```python
from build123d import *

# Parameters (mm, degrees)
EXTRUDE_THIN1_DEPTH          = 10
BOSS_EXTRUDE1_DEPTH          = 2
SKETCH2_W                    = 25.834060226
SKETCH2_H                    = 7.264687176
SKETCH2_W_2                  = 26.707196626
SKETCH2_H_2                  = 6.244092899
CUT_EXTRUDE1_DEPTH           = 92.75076294
SKETCH3_R                    = 4.9
BOSS_EXTRUDE2_DEPTH          = 10
FILLET1_START                = 34.65
FILLET1_DEPTH                = 9.35
FILLET2_R                    = 2
CUT_EXTRUDE2_DEPTH           = 106.894440364
CUT_EXTRUDE2_DEPTH_BACK      = 106.894440364
SKETCH5_R                    = 19.1
SKETCH6_R                    = 2.6162
CUT_EXTRUDE3_DEPTH           = 5
CUT_EXTRUDE3_DRAFT           = -8
CUT_EXTRUDE3_PROFILE_2_DEPTH = 5
CUT_EXTRUDE3_PROFILE_2_DRAFT = -8
CUT_EXTRUDE3_PROFILE_3_DEPTH = 5
CUT_EXTRUDE3_PROFILE_3_DRAFT = -8
CUT_EXTRUDE3_PROFILE_4_DEPTH = 5
CUT_EXTRUDE3_PROFILE_4_DRAFT = -8
SKETCH7_R                    = 2.3495
CUT_EXTRUDE4_DEPTH           = 98.440289419


with BuildPart() as part:
    # Sketch1 → Extrude-Thin1 (new body)
    with BuildSketch(Plane(origin=(0, 32.65, 0), x_dir=(1, 0, 0), z_dir=(0, 1, 0))):
        with BuildLine():
            Line((-69.55, 47.05), (-69.55, -47.05))
            ThreePointArc((-69.55, -47.05), (-66.049926035, -55.499926035), (-57.6, -59))
            Line((-57.6, -59), (-30.4, -59))
            ThreePointArc((-30.4, -59), (-21.950073965, -55.499926035), (-18.45, -47.05))
            Line((-18.45, -47.05), (-18.45, 47.05))
            ThreePointArc((-18.45, 47.05), (-21.950073965, 55.499926035), (-30.4, 59))
            Line((-30.4, 59), (-57.6, 59))
            ThreePointArc((-57.6, 59), (-66.049926035, 55.499926035), (-69.55, 47.05))
        make_face()
        with BuildLine():
            Line((-67.05, 47.05), (-67.05, -47.05))
            ThreePointArc((-67.05, -47.05), (-64.282159082, -53.732159082), (-57.6, -56.5))
            Line((-57.6, -56.5), (-30.4, -56.5))
            ThreePointArc((-30.4, -56.5), (-23.717840918, -53.732159082), (-20.95, -47.05))
            Line((-20.95, -47.05), (-20.95, 47.05))
            ThreePointArc((-20.95, 47.05), (-23.717840918, 53.732159082), (-30.4, 56.5))
            Line((-30.4, 56.5), (-57.6, 56.5))
            ThreePointArc((-57.6, 56.5), (-64.282159082, 53.732159082), (-67.05, 47.05))
        make_face(mode=Mode.SUBTRACT)
    extrude(amount=EXTRUDE_THIN1_DEPTH)

    # Sketch1<2> → Boss-Extrude1 (add)
    with BuildSketch(Plane(origin=(0, 32.65, 0), x_dir=(1, 0, 0), z_dir=(0, 1, 0))):
        with BuildLine():
            Line((-20.95, -47.05), (-20.95, 47.05))
            ThreePointArc((-20.95, 47.05), (-23.717840918, 53.732159082), (-30.4, 56.5))
            Line((-30.4, 56.5), (-57.6, 56.5))
            ThreePointArc((-57.6, 56.5), (-64.282159082, 53.732159082), (-67.05, 47.05))
            Line((-67.05, 47.05), (-67.05, -47.05))
            ThreePointArc((-67.05, -47.05), (-64.282159082, -53.732159082), (-57.6, -56.5))
            Line((-57.6, -56.5), (-30.4, -56.5))
            ThreePointArc((-30.4, -56.5), (-23.717840918, -53.732159082), (-20.95, -47.05))
        make_face()
    extrude(amount=BOSS_EXTRUDE1_DEPTH)

    # Sketch2 → Cut-Extrude1 (cut, through all)
    with BuildSketch(Plane(origin=(0, 42.65, 0), x_dir=(1, 0, 0), z_dir=(0, 1, 0))):
        with Locations((-24.082969887, 60.132343588)):
            Rectangle(SKETCH2_W, SKETCH2_H)
        with Locations((-23.646401687, -59.62204645)):
            Rectangle(SKETCH2_W_2, SKETCH2_H_2)
    extrude(amount=-CUT_EXTRUDE1_DEPTH, mode=Mode.SUBTRACT)

    # Sketch3 → Boss-Extrude2 (add)
    with BuildSketch(Plane(origin=(0, 42.65, 0), x_dir=(1, 0, 0), z_dir=(0, 1, 0))):
        with Locations((-72, -24)):
            Circle(SKETCH3_R)
        with Locations((-16, -32)):
            Circle(SKETCH3_R)
        with Locations((-16, 32)):
            Circle(SKETCH3_R)
        with Locations((-72, 24)):
            Circle(SKETCH3_R)
    extrude(amount=-BOSS_EXTRUDE2_DEPTH)

    # Fillet1: read off the stored shape, not the designer's step
    # Fillet1 outline → Fillet1 (cut)
    with BuildSketch(Plane(origin=(0, 0, 0), x_dir=(1, 0, 0), z_dir=(0, 1, 0)).offset(FILLET1_START)):
        with BuildLine():
            ThreePointArc((-30.4, 56.5), (-27.837508967, 56.145940837), (-25.467033475, 55.110294118))
            ThreePointArc((-25.467033475, 55.110294118), (-25.797428262, 55.953372305), (-25.075528195, 56.5))
            Line((-25.075528195, 56.5), (-30.4, 56.5))
        make_face()
        with BuildLine():
            Line((-30.4, -56.5), (-25.075528195, -56.5))
            ThreePointArc((-25.075528195, -56.5), (-25.797428262, -55.953372305), (-25.467033475, -55.110294118))
            ThreePointArc((-25.467033475, -55.110294118), (-27.837508967, -56.145940837), (-30.4, -56.5))
        make_face()
    extrude(amount=FILLET1_DEPTH, mode=Mode.SUBTRACT)

    # Fillet2
    fillet2_edges = [part.edges().sort_by_distance(p)[0] for p in [
        (-69.55, 37.65, 28.243524479),
        (-69.55, 37.65, 19.756475521),
        (-18.45, 37.65, 27.756475521),
        (-18.45, 37.65, 36.243524479),
        (-18.45, 37.65, -36.243524479),
        (-18.45, 37.65, -27.756475521),
        (-69.55, 37.65, -28.243524479),
        (-69.55, 37.65, -19.756475521),
        (-37, 42.65, -57.75),
        (-37, 42.65, 57.75),
    ]]
    fillet(fillet2_edges, radius=FILLET2_R)

    # Sketch5 → Cut-Extrude2 (cut, two sides: drawn at the far end of the back side and taken through both)
    with BuildSketch(Plane.XY.offset(-CUT_EXTRUDE2_DEPTH_BACK)):
        with Locations((0, 55.15)):
            Circle(SKETCH5_R)
    extrude(amount=CUT_EXTRUDE2_DEPTH + CUT_EXTRUDE2_DEPTH_BACK, mode=Mode.SUBTRACT)


with BuildPart() as cut_extrude3_tool:
    # Sketch6 → Cut-Extrude3 (with draft: the straight prism first)
    with BuildSketch(Plane.XZ.offset(-32.65)):
        with Locations((-72, 24)):
            Circle(SKETCH6_R)
    extrude(amount=-CUT_EXTRUDE3_DEPTH)
    # Cut-Extrude3: the draft: its side faces are tilted about the plane it starts from
    cut_extrude3_sides = [cut_extrude3_tool.faces().sort_by_distance(p)[0] for p in [
        (-74.6162, 35.15, 24),
    ]]
    draft(cut_extrude3_sides, Plane.XZ.offset(-32.65), CUT_EXTRUDE3_DRAFT)


with BuildPart() as part_1:
    add(part.part)

    # Cut-Extrude3: cut by cut_extrude3_tool
    add(cut_extrude3_tool.part, mode=Mode.SUBTRACT)


with BuildPart() as cut_extrude3_profile_2_tool:
    # Sketch6 → Cut-Extrude3 profile 2 (with draft: the straight prism first)
    with BuildSketch(Plane.XZ.offset(-32.65)):
        with Locations((-16, 32)):
            Circle(SKETCH6_R)
    extrude(amount=-CUT_EXTRUDE3_PROFILE_2_DEPTH)
    # Cut-Extrude3 profile 2: the draft: its side faces are tilted about the plane it starts from
    cut_extrude3_profile_2_sides = [cut_extrude3_profile_2_tool.faces().sort_by_distance(p)[0] for p in [
        (-18.6162, 35.15, 32),
    ]]
    draft(cut_extrude3_profile_2_sides, Plane.XZ.offset(-32.65), CUT_EXTRUDE3_PROFILE_2_DRAFT)


with BuildPart() as part_2:
    add(part_1.part)

    # Cut-Extrude3 profile 2: cut by cut_extrude3_profile_2_tool
    add(cut_extrude3_profile_2_tool.part, mode=Mode.SUBTRACT)


with BuildPart() as cut_extrude3_profile_3_tool:
    # Sketch6 → Cut-Extrude3 profile 3 (with draft: the straight prism first)
    with BuildSketch(Plane.XZ.offset(-32.65)):
        with Locations((-16, -32)):
            Circle(SKETCH6_R)
    extrude(amount=-CUT_EXTRUDE3_PROFILE_3_DEPTH)
    # Cut-Extrude3 profile 3: the draft: its side faces are tilted about the plane it starts from
    cut_extrude3_profile_3_sides = [cut_extrude3_profile_3_tool.faces().sort_by_distance(p)[0] for p in [
        (-18.6162, 35.15, -32),
    ]]
    draft(cut_extrude3_profile_3_sides, Plane.XZ.offset(-32.65), CUT_EXTRUDE3_PROFILE_3_DRAFT)


with BuildPart() as part_3:
    add(part_2.part)

    # Cut-Extrude3 profile 3: cut by cut_extrude3_profile_3_tool
    add(cut_extrude3_profile_3_tool.part, mode=Mode.SUBTRACT)


with BuildPart() as cut_extrude3_profile_4_tool:
    # Sketch6 → Cut-Extrude3 profile 4 (with draft: the straight prism first)
    with BuildSketch(Plane.XZ.offset(-32.65)):
        with Locations((-72, -24)):
            Circle(SKETCH6_R)
    extrude(amount=-CUT_EXTRUDE3_PROFILE_4_DEPTH)
    # Cut-Extrude3 profile 4: the draft: its side faces are tilted about the plane it starts from
    cut_extrude3_profile_4_sides = [cut_extrude3_profile_4_tool.faces().sort_by_distance(p)[0] for p in [
        (-74.6162, 35.15, -24),
    ]]
    draft(cut_extrude3_profile_4_sides, Plane.XZ.offset(-32.65), CUT_EXTRUDE3_PROFILE_4_DRAFT)


with BuildPart() as part_4:
    add(part_3.part)

    # Cut-Extrude3 profile 4: cut by cut_extrude3_profile_4_tool
    add(cut_extrude3_profile_4_tool.part, mode=Mode.SUBTRACT)

    # Sketch7 → Cut-Extrude4 (cut, through all)
    with BuildSketch(Plane.XZ.offset(-32.65)):
        with Locations(Location((-72, 24, 0), (0, 0, 270))):
            Circle(SKETCH7_R)
        with Locations(Location((-16, 32, 0), (0, 0, 270))):
            Circle(SKETCH7_R)
        with Locations(Location((-16, -32, 0), (0, 0, 270))):
            Circle(SKETCH7_R)
        with Locations(Location((-72, -24, 0), (0, 0, 270))):
            Circle(SKETCH7_R)
    extrude(amount=-CUT_EXTRUDE4_DEPTH, mode=Mode.SUBTRACT)


solid = part_4.part
```
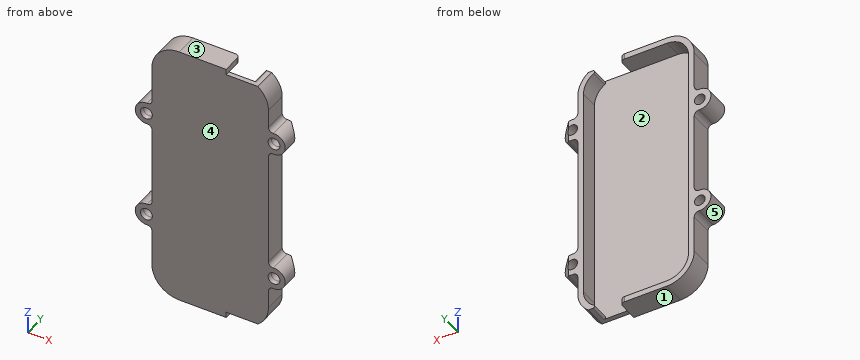
The listing builds one solid part. Answer for the finished solid, in the listing's coordinates (mm). Face numbers are marked on the shaded views. A direction names the side the tool comes from. Round coordinates to 2 decimals unless told otherwise and drop trailing zeros. Order: outer loops, then holes, each group sorted by start corner. A loop starts at its lowest first (then second) coordinate and runs counter-clockwise, first axis right, second up. Notation, with made-up numbers: (29.5, 2) - (58.5, 2) arc R23 cw to (58.5, 29) - close; hole circle Ø6 at (35.25, -5). An arc over 180 degrees is marked (long way). Put each result on its own line as item: value. Start each with the question number.
(1) Find section D-D (y = 38.25). State how many separate pieces and enclosed holes the cut face has, plus the area to 3 significant figures.
(2) Find section C-C (x = -62.5). Give the vertices of the cut face in (y, z).
(3) Given P1, Ø2, axis at x = -66, y = 37.5, coming from the -Z side; P2, Ø5, axis at x = -30.5, y = 36.5, coming from the +Z side; P3, Ø3, axis at x = -61, z = 37.5, coming from the +Y side, each flat-ended and moving along its own axis, determine where each tip first touches the part or whether it passes through.
(4) For the marked faces 1 and 2, determine the directions among +Z, -Z, +X, -X, +Y, -Y from which every point of the face is accessible in a straight line to the end or side of a thin tool.
(5) Determine the mould class of the marked faces 3, 4 and 5 for opening direction Z: released by +Z, released by -Z, zero draft, split by the parting line, or undercut.
(6) Straight lines are drawn through the part: probe 1 along Z at (x, y) = (-72, 36.5); probe 2 along Z at (x, y) = (-16, 40.5); probe 3 along X at (y, z) = (37.25, -3.5). For each, find the intervals that lie inside material, in ascending order. Write a range as from..to.
(7) Find section A-A (z = -24). Give the vertices of the cut face in (x, y).
(8) Find section B-B (z = -2.5). Give the vertices of the cut face in (x, y), plus the area to 3 significant figures.
Reply:
1. separate pieces: 2
1. enclosed holes: 4
1. area: 897 mm^2
2. outline: (32.65, -57.95) - (42.65, -57.95) - (42.65, -55.13) - (34.65, -55.13) - (34.65, 55.13) - (42.65, 55.13) - (42.65, 57.95) - (32.65, 57.95) - close
3. P1: z = -56.43
3. P2: z = 56.5
3. P3: y = 34.65
4. face 1: -Z, +X, -X, +Y, -Y
4. face 2: +Y
5. face 3: released by +Z
5. face 4: zero draft
5. face 5: undercut
6. probe 1: -28.9..-26.35, -21.65..-19.1, 19.1..21.65, 26.35..28.9
6. probe 2: -36.9..-34.35, -29.65..-27.1, 27.1..29.65, 34.35..36.9
6. probe 3: -69.55..-67.05, -20.95..-18.45
7. outline: (-76.9, 32.65) - (-74.62, 32.65) - (-74.35, 34.55) - (-74.35, 42.65) - (-76.9, 42.65) - close; (-69.65, 34.55) - (-69.38, 32.65) - (-18.45, 32.65) - (-18.45, 42.65) - (-20.95, 42.65) - (-20.95, 34.65) - (-67.05, 34.65) - (-67.05, 42.65) - (-69.65, 42.65) - close
8. outline: (-69.55, 32.65) - (-18.45, 32.65) - (-18.45, 42.65) - (-20.95, 42.65) - (-20.95, 34.65) - (-67.05, 34.65) - (-67.05, 42.65) - (-69.55, 42.65) - close
8. area: 142 mm^2
